Could you check a few things on this drawing? It's one solid part, dimensions in mm from its lowest x, y, z. A direction names the side the tool comes from. Give positions to 0.01 mm unless a question says otherwise; leave off trailing zeros. Order: outer loops, then holes, each group sorted by start corner. A loop starts at its lowest first (then second) coordinate and runs counter-clockwise, first axis right, second up.
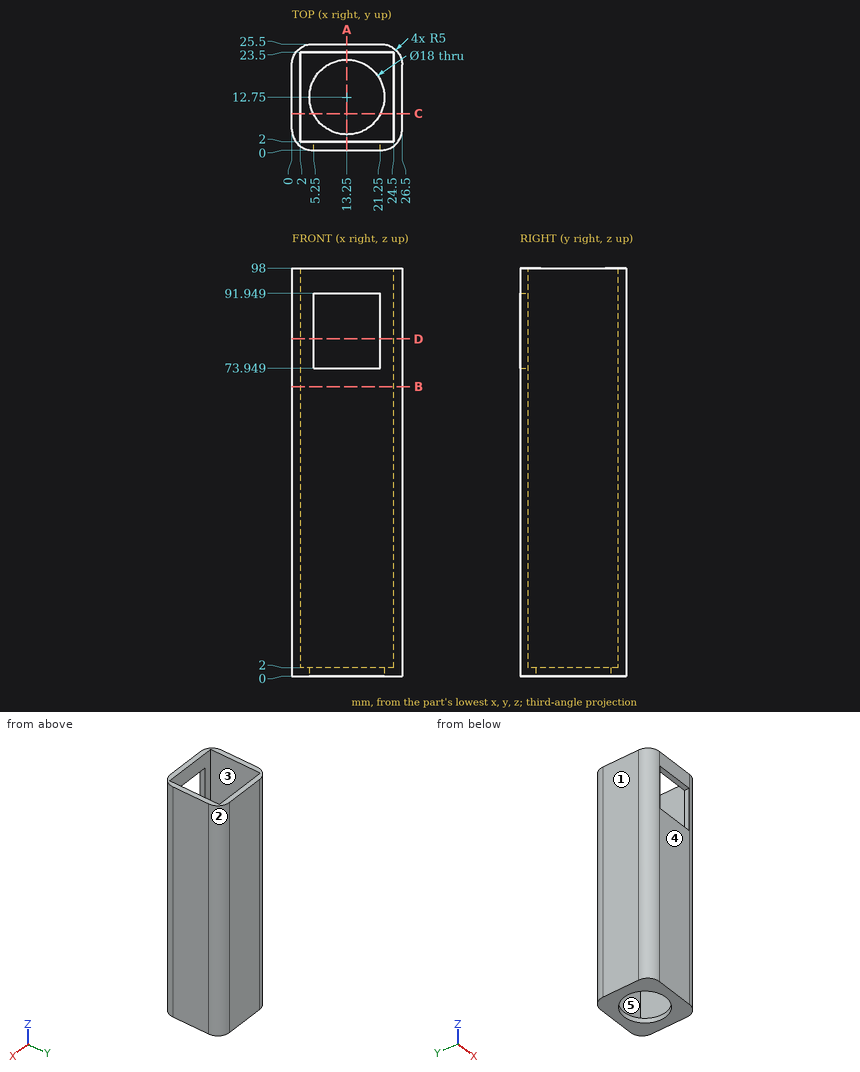
Q1. I need wall thicknesses on L1, parallel to X at y = 10.5, z = 31.5; L2, parallel to Z at x = 7, y = 1.25; L3, parallel to Y at x = 13.25, z = 0.8. Which ranges of each line are inside material? Lowest first, please.
Filled sheet:
L1: x = 0 to 2, 24.5 to 26.5
L2: z = 0 to 73.95, 91.95 to 98
L3: y = 0 to 3.75, 21.75 to 25.5
Q2. Thinking about a two-plate mould opening in X: for the marked faces 1, 2 and 3, which applies, released by +X, released by -X, zero draft, split by the parting line, or undercut?
Filled sheet:
face 1: released by -X
face 2: released by +X
face 3: undercut
Q3. If we section it at C-C on y = 8.75: List the corners of the cut face in (x, z) for me.
Filled sheet:
outline: (0, 0) - (5.19, 0) - (5.19, 2) - (2, 2) - (2, 98) - (0, 98) - close; (21.31, 0) - (26.5, 0) - (26.5, 98) - (24.5, 98) - (24.5, 2) - (21.31, 2) - close
Q4. I'm going to push flat-ended pins straight in: P1, Ø1, axis at y = 3, z = 44, coming from the +X side; P2, Ø3, axis at x = 6.5, y = 20, coming from the +Z side; P3, Ø0.6, axis at y = 1.5, z = 80, coming from the -X side. Where does each tip first touch, or does it pass through?
Filled sheet:
P1: stops at x = 26.27
P2: stops at z = 2
P3: stops at x = 1.16
Q5. For the marked faces 4 and 5, which set-ups out of +Z, -Z, +X, -X, +Y, -Y let a thin tool reach every point of the face, with its end or its side?
Filled sheet:
face 4: +Z, -Z, +X, -X, -Y
face 5: +Z
Q6. If we section it at B-B on z = 69.5: List the corners of the cut face in (x, y) for me.
Filled sheet:
outline: (0, 5) arc R5 ccw to (5, 0) - (21.5, 0) arc R5 ccw to (26.5, 5) - (26.5, 20.5) arc R5 ccw to (21.5, 25.5) - (5, 25.5) arc R5 ccw to (0, 20.5) - close; hole (2, 2) - (24.5, 2) - (24.5, 23.5) - (2, 23.5) - close
Q7. If we section it at D-D on z = 81: List the corners of the cut face in (x, y) for me.
Filled sheet:
outline: (0, 5) arc R5 ccw to (5, 0) - (5.25, 0) - (5.25, 2) - (2, 2) - (2, 23.5) - (24.5, 23.5) - (24.5, 2) - (21.25, 2) - (21.25, 0) - (21.5, 0) arc R5 ccw to (26.5, 5) - (26.5, 20.5) arc R5 ccw to (21.5, 25.5) - (5, 25.5) arc R5 ccw to (0, 20.5) - close
Q8. If we section it at A-A on x = 13.25: List the corners of the cut face in (y, z) for me.
Filled sheet:
outline: (0, 0) - (3.75, 0) - (3.75, 2) - (2, 2) - (2, 73.95) - (0, 73.95) - close; (0, 91.95) - (2, 91.95) - (2, 98) - (0, 98) - close; (21.75, 0) - (25.5, 0) - (25.5, 98) - (23.5, 98) - (23.5, 2) - (21.75, 2) - close
